Geometry check sheet. Reference: the model listing, model coordinates, mm. Face numbers are marked on the shaded views. A direction names the side the tool comes from. Round coordinates to 2 decimals unless told otherwise and drop trailing zeros. Write each loop counter-clockwise with the first axis right and the second up, starting at its lowest first coordinate (ties: lowest second). Pieces come first, ordered by that corner, then holes.
Item 1: Scan lines: probe 1 along Z at (x, y) = (15, 21) (3 decimals); probe 2 along Y at (x, z) = (6.25, -8.75) (3 decimals); probe 3 along Y at (x, z) = (19.5, -26.5). Record each from-to range of solid material in increasing order.
Item 2: Depth check by flat-ended pin: P1, Ø2, axis at x = 14, y = 12, coming from the +Z side; P2, Ø1, axis at x = 9.5, z = -15, coming from the +Y side (3 decimals). Enter the tip coordinate at first touch or a pass-through.
Item 3: Cross-section at D-D (x = 2.75). Enter the section's corners in (y, z) (3 decimals), then the cut area to 3 significant figures.
Item 4: Cross-section at C-C (z = -20.75). Enter the section's corners in (x, y) (3 decimals).
Item 5: Cross-section at B-B (y = 5.25). Enter the section's corners in (x, z) (3 decimals).
Item 6: Access from +Z, -Z, +X, -X, +Y, -Y to the whole of each face (thin tool, end or side, straight path). Record for the marked faces 1 and 2.
Item 7: Cross-section at A-A (x = 9.25). Enter the section's corners in (y, z) (3 decimals).
from build123d import *

# Parameters (mm, degrees)
SKETCH2_W               = 25.4
SKETCH2_H               = 28.175
BOSS_EXTRUDE1_DEPTH     = 3.175
SKETCH3_W               = 25.4
SKETCH3_H               = 3.175
BOSS_EXTRUDE2_DEPTH     = 25
CUT_EXTRUDE1_DEPTH      = 26
CUT_EXTRUDE1_DEPTH_BACK = 4.175


with BuildPart() as part:
    # Sketch2 → Boss-Extrude1 (new body)
    with BuildSketch(Plane(origin=(0, 0, 0), x_dir=(1, 0, 0), z_dir=(0, 1, 0))):
        with Locations((12.7, 14.0875)):
            Rectangle(SKETCH2_W, SKETCH2_H)
    extrude(amount=BOSS_EXTRUDE1_DEPTH)

    # Sketch3 → Boss-Extrude2 (add)
    with BuildSketch(Plane(origin=(0, 3.175, 0), x_dir=(1, 0, 0), z_dir=(0, 1, 0))):
        with Locations((12.7, 26.5875)):
            Rectangle(SKETCH3_W, SKETCH3_H)
    extrude(amount=BOSS_EXTRUDE2_DEPTH)

    # Sketch4 → Cut-Extrude1 (cut, two sides)
    with BuildSketch(Plane.XY.offset(-25)) as cut_extrude1_sk:
        Polygon((-36.811931354, -69.289431798), (0, 3.175), (12.7, 28.175), (25.4, 3.175), (62.211931354, -69.289431798), (62.211931354, 93.267784785), (-36.811931354, 93.267784785), align=None)
    extrude(amount=CUT_EXTRUDE1_DEPTH, mode=Mode.SUBTRACT)
    extrude(cut_extrude1_sk.sketch, amount=-CUT_EXTRUDE1_DEPTH_BACK, mode=Mode.SUBTRACT)


solid = part.part
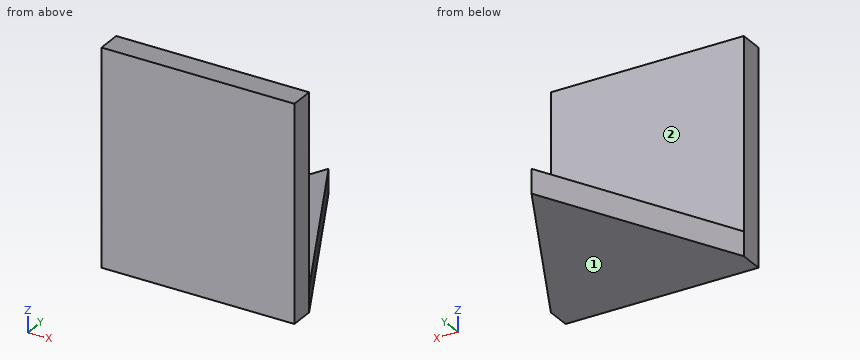
Resolved:
1. probe 1: z = -28.175 to -25
1. probe 2: y = 0 to 3.175
1. probe 3: y = 0 to 14.79
2. P1: stops at z = -25
2. P2: stops at y = 3.175
3. outline: (0, -28.175) - (8.588, -28.175) - (8.588, -25) - (3.175, -25) - (3.175, 0) - (0, 0) - close
3. area: 107 mm2
4. outline: (0, 0) - (25.4, 0) - (25.4, 3.175) - (0, 3.175) - close
5. outline: (1.054, -28.175) - (24.346, -28.175) - (24.346, -25) - (1.054, -25) - close
6. face 1: -Z, +X, -X, +Y, -Y
6. face 2: +Z, +X, -X, +Y
7. outline: (0, -28.175) - (21.384, -28.175) - (21.384, -25) - (3.175, -25) - (3.175, 0) - (0, 0) - close
